Here's how the part is built. I have some questions about the finished solid (model axes, mm). A direction names the side the tool comes from. Round coordinates to 2 decimals unless told otherwise and drop trailing zeros. Write each loop counter-clockwise with the first axis right and the second up, starting at its lowest first coordinate (ties: lowest second). Pieces come first, ordered by that corner, then holes. Notation, with made-up numbers: (63.5, 53.25) -> (121.5, 53.25) arc R14 cw to (121.5, 60.25) -> close; hole circle Ø8 at (89.5, 8). An arc over 180 degrees is marked (long way). Put each result on its own line as item: value. Start each with the question number.
1. Suppose I cut it at C-C (x = 8). Please give me the cut outline in (y, z), then the cut area to 3 significant figures.
2. Suppose I cut it at B-B (z = 2.7). Please give me the cut outline in (x, y), then the cut area to 3 significant figures.
3. For pin 1 (4 mm diameter, centred on x = 3.75, y = 2, fed in from -Z); pin 2 (2 mm diameter, centred on x = 7.5, z = 3, fed in from +Y), each with a flat end and sliding along its axis, tell me the tip position at first contact or that it passes through.
4. We'd pull the mould along X, two halves only. Please class faces 4 (the face through (26.64, 2.46, 2.55)), 5 (the face through (0.57, 0.6, 2.06)), 6 (the face through (54.93, 66.1, 2.06)): +X half, -X half, draft (parallel to the pull), parting line (faces both ways), or undercut.
5. I need wall thicknesses on probe 1 along X at (y, z) = (64.7, 2.7); probe 2 along Y at (x, z) = (3.75, 2.35); probe 3 along Y at (x, z) = (29, 0.7). Which ranges of each line are inside material? Lowest first, please. Write a range as from..to.
6. Suppose I cut it at A-A (x = 27.75). Please give me the cut outline in (y, z).
7. Which directions (+Z, -Z, +X, -X, +Y, -Y) give clear straight access to the entire face, cutting with the end or side of a thin tool? Please do faces 1 (the face through (27, 0, 2)), 2 (the face through (28, 66.7, 2)), 3 (the face through (6, 66.7, 2)).
```python
from build123d import *

# Parameters (mm, degrees)
SKETCH1_W                                       = 55.5
SKETCH1_H                                       = 66.7
BOSS_EXTRUDE1_DEPTH                             = 4.064
CSK_FOR_M2_FLAT_HEAD_MACHINE_SCREW3_D           = 2.4
CSK_FOR_M2_FLAT_HEAD_MACHINE_SCREW3_CSINK_D     = 4.4
CSK_FOR_M2_FLAT_HEAD_MACHINE_SCREW3_CSINK_ANGLE = 90
FILLET1_R                                       = 2
BOSS_EXTRUDE3_DEPTH                             = 4.064
FILLET2_R                                       = 1


with BuildPart() as part:
    # Sketch1 → Boss-Extrude1 (new body)
    with BuildSketch(Plane.XY):
        with Locations((27.75, 33.35)):
            Rectangle(SKETCH1_W, SKETCH1_H)
    extrude(amount=BOSS_EXTRUDE1_DEPTH)

    # CSK for M2 Flat Head Machine Screw3 (through all)
    with Locations(Plane(origin=(2.783474674, 10.392611329, 0), x_dir=(1, 0, 0), z_dir=(0, 0, -1))):
        with Locations((0.966525326, -54.307388671), (24.966525326, -54.307388671), (48.966525326, -54.307388671), (0.966525326, 8.392611329), (24.966525326, 8.392611329), (48.966525326, 8.392611329)):
            CounterSinkHole(CSK_FOR_M2_FLAT_HEAD_MACHINE_SCREW3_D / 2, CSK_FOR_M2_FLAT_HEAD_MACHINE_SCREW3_CSINK_D / 2, counter_sink_angle=CSK_FOR_M2_FLAT_HEAD_MACHINE_SCREW3_CSINK_ANGLE)

    # Fillet1
    fillet1_edges = [part.edges().sort_by_distance(p)[0] for p in [
        (0, 66.7, 2.032),
        (55.5, 66.7, 2.032),
        (55.5, 0, 2.032),
        (0, 0, 2.032),
    ]]
    fillet(fillet1_edges, radius=FILLET1_R)

    # Sketch7 → Boss-Extrude3 (add, through all)
    with BuildSketch(Plane.XY.offset(4.064)):
        with BuildLine():
            Line((10.25, 66.7), (13.25, 66.7))
            ThreePointArc((13.25, 66.7), (11.75, 68.2), (10.25, 66.7))
        make_face()
        with BuildLine():
            Line((42.25, 66.7), (45.25, 66.7))
            ThreePointArc((45.25, 66.7), (43.75, 68.2), (42.25, 66.7))
        make_face()
    extrude(amount=-BOSS_EXTRUDE3_DEPTH)

    # Fillet2
    fillet2_edges = [part.edges().sort_by_distance(p)[0] for p in [
        (10.25, 66.7, 2.032),
        (13.25, 66.7, 2.032),
        (42.25, 66.7, 2.032),
        (45.25, 66.7, 2.032),
    ]]
    fillet(fillet2_edges, radius=FILLET2_R)


solid = part.part
```
Verdict:
1. outline: (0, 0) -> (66.7, 0) -> (66.7, 4.06) -> (0, 4.06) -> close
1. area: 271 mm^2
2. outline: (0, 2) arc R2 ccw to (2, 0) -> (53.5, 0) arc R2 ccw to (55.5, 2) -> (55.5, 64.7) arc R2 ccw to (53.5, 66.7) -> (46.04, 66.7) arc R1 cw to (45.12, 67.3) arc R1.5 ccw to (42.38, 67.3) arc R1 cw to (41.46, 66.7) -> (14.04, 66.7) arc R1 cw to (13.12, 67.3) arc R1.5 ccw to (10.38, 67.3) arc R1 cw to (9.46, 66.7) -> (2, 66.7) arc R2 ccw to (0, 64.7) -> close; hole circle Ø2.4 at (3.75, 2); hole circle Ø2.4 at (3.75, 64.7); hole circle Ø2.4 at (27.75, 2); hole circle Ø2.4 at (27.75, 64.7); hole circle Ø2.4 at (51.75, 2); hole circle Ø2.4 at (51.75, 64.7)
2. area: 3,680 mm^2
3. pin 1: stops at z = 0.2
3. pin 2: stops at y = 66.7
4. face 4: undercut
4. face 5: -X half
4. face 6: +X half
5. probe 1: x = 0..2.55, 4.95..26.55, 28.95..50.55, 52.95..55.5
5. probe 2: y = 0..0.8, 3.2..63.5, 65.9..66.7
5. probe 3: y = 0..1.17, 2.83..63.87, 65.53..66.7
6. outline: (0, 0.2) -> (0.8, 1) -> (0.8, 4.06) -> (0, 4.06) -> close; (3.2, 1) -> (4.2, 0) -> (62.5, 0) -> (63.5, 1) -> (63.5, 4.06) -> (3.2, 4.06) -> close; (65.9, 1) -> (66.7, 0.2) -> (66.7, 4.06) -> (65.9, 4.06) -> close
7. face 1: +Z, -Z, +X, -X, -Y
7. face 2: +Z, -Z, +Y
7. face 3: +Z, -Z, -X, +Y
